Model file for the job. Use its own axes, mm. Face numbers are marked on the shaded views. A direction names the side the tool comes from. Give positions to 0.01 mm unless a question says otherwise; leave off trailing zeros. Order: outer loops, then holes, each group sorted by start corner. A loop starts at its lowest first (then second) coordinate and runs counter-clockwise, first axis right, second up. Notation, with made-up numbers: M 9,-16 L 13,-16 A13 cw 13,7 Z; hole C 47.5,21 d2. An arc over 180 degrees is marked long. Return JSON: item names as keys, results as strings. Group by question number.
1. Slice it at C-C on y = 36.5. List the corners of the cut face in (x, z), then the cut area to 3 significant figures.
2. Wall check: probe 1 along X at (y, z) = (2, -52.5); probe 2 along X at (y, z) = (1, -29); probe 3 along Y at (x, z) = (18.5, -15). Give the ranges that are in metal, low to high. Write a range as [from, to].
3. Slice it at A-A on z = -52.5. List the corners of the cut face in (x, y).
4. 3-axis set-ups, long thin cutter, end or side, ignore diameter. For the marked faces 4 and 5: which of +Z, -Z, +X, -X, +Y, -Y reach the whole face in a straight line?
5. Slice it at D-D on x = -15. List the corners of the cut face in (y, z) (3 decimals), then the cut area to 3 significant figures.
6. Slice it at B-B on z = -29. List the corners of the cut face in (x, y).
7. Pin check, flat tips, straight feed: pin 1 (4.5 mm diameter, centred on x = 23.5, z = -52.5, fed in from +Y); pin 2 (12 mm diameter, centred on y = 11.5, z = -51, fed in from -X); pin 3 (6 mm diameter, centred on x = -11, z = -58.5, fed in from +Y); pin 4 (6 mm diameter, centred on x = -7.5, y = 10.5, fed in from +Z). Stop position of each tip, or through.
8. Two-plate mould, pull along X, no slides. Class the marked faces 1, 2 and 3: released by +X, released by -X, zero draft, split by the parting line, or undercut.
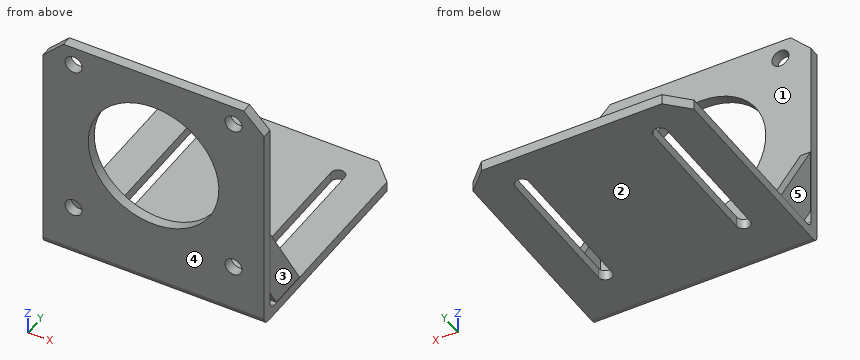
from build123d import *

# Parameters (mm, degrees)
SKETCH1_W           = 65
SKETCH1_H           = 65
BOSS_EXTRUDE1_DEPTH = 3
SKETCH2_W           = 65
SKETCH2_H           = 3
BOSS_EXTRUDE2_DEPTH = 68
SKETCH4_R           = 19.2
CUT_EXTRUDE1_DEPTH  = 100.525122457
SKETCH5_R           = 2.5
CUT_EXTRUDE2_DEPTH  = 100.525122457
CUT_EXTRUDE3_DEPTH  = 100.525122457
BOSS_EXTRUDE3_START = -0.1
BOSS_EXTRUDE3_DEPTH = 3
BOSS_EXTRUDE4_START = -0.1
BOSS_EXTRUDE4_DEPTH = 3
FILLET1_R           = 2
CHAMFER1_SIZE       = 6


with BuildPart() as part:
    # Sketch1 → Boss-Extrude1 (new body)
    with BuildSketch(Plane(origin=(0, 0, 0), x_dir=(1, 0, 0), z_dir=(0, 1, 0))):
        with Locations((0, 32.5)):
            Rectangle(SKETCH1_W, SKETCH1_H)
    extrude(amount=BOSS_EXTRUDE1_DEPTH)

    # Sketch2 → Boss-Extrude2 (add)
    with BuildSketch(Plane.XZ):
        with Locations((0, -66.5)):
            Rectangle(SKETCH2_W, SKETCH2_H)
    extrude(amount=-BOSS_EXTRUDE2_DEPTH)

    # Sketch4 → Cut-Extrude1 (cut, through all)
    with BuildSketch(Plane(origin=(0, 3, 0), x_dir=(1, 0, 0), z_dir=(0, 1, 0))):
        with Locations(Location((0, 29, 0), (0, 0, 270))):
            Circle(SKETCH4_R)
    extrude(amount=-CUT_EXTRUDE1_DEPTH, mode=Mode.SUBTRACT)

    # Sketch5 → Cut-Extrude2 (cut, through all)
    with BuildSketch(Plane(origin=(0, 3, 0), x_dir=(1, 0, 0), z_dir=(0, 1, 0))):
        with Locations(Location((-23.5, 52.5, 0), (0, 0, 270))):
            Circle(SKETCH5_R)
        with Locations(Location((23.5, 52.5, 0), (0, 0, 270))):
            Circle(SKETCH5_R)
        with Locations(Location((23.5, 5.5, 0), (0, 0, 270))):
            Circle(SKETCH5_R)
        with Locations(Location((-23.5, 5.5, 0), (0, 0, 270))):
            Circle(SKETCH5_R)
    extrude(amount=-CUT_EXTRUDE2_DEPTH, mode=Mode.SUBTRACT)

    # Sketch6 → Cut-Extrude3 (cut, through all)
    with BuildSketch(Plane.XY.offset(-65)):
        with BuildLine():
            Line((-18.3, 58.2), (-18.3, 16.2))
            ThreePointArc((-18.3, 16.2), (-20.3, 14.2), (-22.3, 16.2))
            Line((-22.3, 16.2), (-22.3, 58.2))
            ThreePointArc((-22.3, 58.2), (-20.3, 60.2), (-18.3, 58.2))
        make_face()
        with BuildLine():
            Line((18.3, 58.2), (18.3, 16.2))
            ThreePointArc((18.3, 16.2), (20.3, 14.2), (22.3, 16.2))
            Line((22.3, 16.2), (22.3, 58.2))
            ThreePointArc((22.3, 58.2), (20.3, 60.2), (18.3, 58.2))
        make_face()
    extrude(amount=-CUT_EXTRUDE3_DEPTH, mode=Mode.SUBTRACT)

    # Sketch8 → Boss-Extrude3 (add)
    with BuildSketch(Plane.ZY.offset(32.5).offset(BOSS_EXTRUDE3_START)):
        Polygon((-40, 3), (-65, 18), (-65, 6.33809621), (-59.436506316, 3), align=None)
    extrude(amount=-BOSS_EXTRUDE3_DEPTH)

    # Sketch9 → Boss-Extrude4 (add)
    with BuildSketch(Plane(origin=(32.5, 0, 0), x_dir=(0, 0, -1), z_dir=(1, 0, 0)).offset(BOSS_EXTRUDE4_START)):
        Polygon((40, 3), (59.436506316, 3), (65, 6.33809621), (65, 18), align=None)
    extrude(amount=-BOSS_EXTRUDE4_DEPTH)

    # Fillet1
    fillet1_edges = [part.edges().sort_by_distance(p)[0] for p in [
        (0, 3, -65),
        (0, 0, -68),
    ]]
    fillet(fillet1_edges, radius=FILLET1_R)

    # Chamfer1
    chamfer1_edges = [part.edges().sort_by_distance(p)[0] for p in [
        (-32.5, 68, -66.5),
        (32.5, 68, -66.5),
        (32.5, 1.5, 0),
        (-32.5, 1.5, 0),
    ]]
    chamfer(chamfer1_edges, length=CHAMFER1_SIZE)


solid = part.part
Result:
{
 "1": {"outline": "M -32.5,-68 L -22.3,-68 L -22.3,-65 L -32.5,-65 Z; M -18.3,-68 L 18.3,-68 L 18.3,-65 L -18.3,-65 Z; M 22.3,-68 L 32.5,-68 L 32.5,-65 L 22.3,-65 Z", "area": "171 mm2"},
 "2": {"probe 1": "x = [-32.5, -26], [-21, 21], [26, 32.5]", "probe 2": "x = [-32.5, -19.2], [19.2, 32.5]", "probe 3": "y = [0, 3]"},
 "3": {"outline": "M -32.5,0 L -26,0 L -26,3 L -29.4,3 L -29.4,10.5 L -32.4,10.5 L -32.4,3 L -32.5,3 Z; M -21,0 L 21,0 L 21,3 L -21,3 Z; M 26,0 L 32.5,0 L 32.5,3 L 32.4,3 L 32.4,10.5 L 29.4,10.5 L 29.4,3 L 26,3 Z"},
 "4": {"face 4": "+Z, -Z, +X, -X, -Y", "face 5": "+Z, -X, +Y"},
 "5": {"outline": "M 0,-66 A2 ccw 2,-68 L 68,-68 L 68,-65 L 5,-65 A2 cw 3,-63 L 3,-40.985 L 0,-40.985 Z; M 0,-17.015 L 3,-17.015 L 3,0 L 0,0 Z", "area": "327 mm2"},
 "6": {"outline": "M -32.5,0 L -19.2,0 L -19.2,3 L -32.5,3 Z; M 19.2,0 L 32.5,0 L 32.5,3 L 19.2,3 Z"},
 "7": {"pin 1": "passes through", "pin 2": "stops at x = -32.4", "pin 3": "stops at y = 3", "pin 4": "stops at z = -65"},
 "8": {"face 1": "undercut", "face 2": "zero draft", "face 3": "released by +X"}
}
